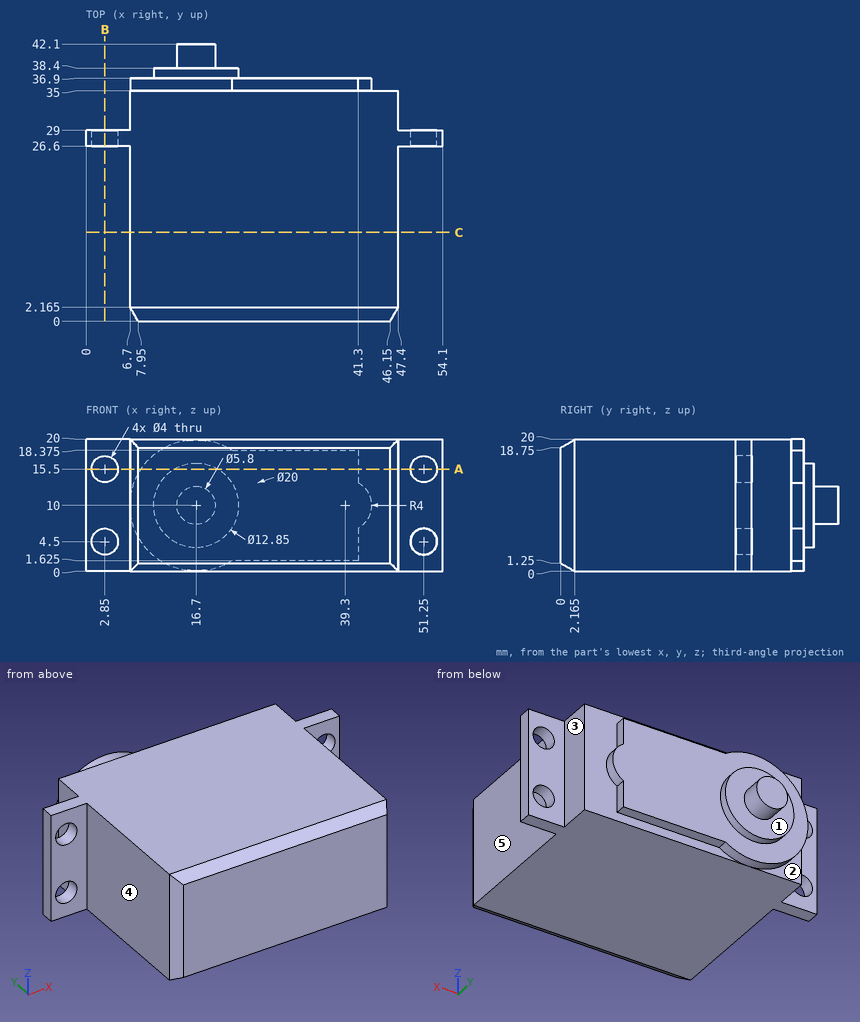
Geometry check sheet. Reference: drawing and pictorial views, mm from the part's lowest x, y, z. A direction names the side the tool comes from. Round coordinates to 2 decimals unless told otherwise and drop trailing zeros. Order: outer loops, then holes, each group sorted by start corner. A loop starts at its lowest first (then second) coordinate and runs counter-clockwise, first axis right, second up. Notation, with made-up numbers: M 2.5,-31 L 31.5,-31 A13 ccw 31.5,-18 Z; hole C -13.5,88 d2. An arc over 180 degrees is marked long. One line per item, written item: value. Start each with the question number.
1. Access from +Z, -Z, +X, -X, +Y, -Y to the whole of each face (thin tool, end or side, straight path). Record for the marked faces 1, 2, 3, 4 and 5.
2. Scan lines: line 1 along X through (y, z) = (27.95, 15.5); line 2 along X through (y, z) = (8, 6.75); line 3 along Y through (x, z) = (10.5, 10). Record each from-to range of solid material in increasing order.
3. Section check A-A on z = 15.5. Give the number of separate pieces and of enclosed holes in the cut face, and give its area (3 significant figures).
4. Gauge pin test, flat ends, axial feed: P1, Ø5.5, axis at x = 49.5, z = 5.5, coming from the -Y side; P2, Ø4.5, axis at x = 2.85, z = 15.5, coming from the +Y side; P3, Ø5, axis at y = 35, z = 8, coming from the +X side. Record the tip position at first contact, or that the pin passes through.
5. Section check B-B on x = 2.85. Enter the section's corners in (y, z).
6. Section check C-C on y = 13.5. Enter the section's corners in (x, z), and give its area (3 significant figures).
Results found:
1. face 1: +Y
1. face 2: -Z, -X, +Y
1. face 3: +Z, -Z, +X, +Y
1. face 4: +Z, -Z, -X, -Y
1. face 5: +Z, -Z, +X, -Y
2. line 1: 0 to 0.85, 4.85 to 49.25, 53.25 to 54.1
2. line 2: 6.7 to 47.4
2. line 3: 0 to 38.4
3. separate pieces: 3
3. enclosed holes: 0
3. area: 1,510 mm^2
4. P1: y = 1.04
4. P2: y = 29
4. P3: x = 47.4
5. outline: M 26.6,0 L 29,0 L 29,2.5 L 26.6,2.5 Z; M 26.6,6.5 L 29,6.5 L 29,13.5 L 26.6,13.5 Z; M 26.6,17.5 L 29,17.5 L 29,20 L 26.6,20 Z
6. outline: M 6.7,0 L 47.4,0 L 47.4,20 L 6.7,20 Z
6. area: 814 mm^2
